Autodesk Inventor part; units mm, degrees
ref_plane "YZ Plane" through (0, 0, 0) normal (1, 0, 0) x (0, 1, 0)
ref_plane "XZ Plane" through (0, 0, 0) normal (0, 1, 0) x (-1, 0, 0)
ref_plane "XY Plane" through (0, 0, 0) normal (0, 0, 1) x (1, 0, 0)
sketch "Sketch1" plane through (0, 0, 0) normal (0, 0, 1) x (1, 0, 0)
  arc A0 (155.049, 9.8568) -> (142.3409, 9.8568) centre (148.6949, 9.8608) ccw
  circle A1 centre (148.6949, 9.8568) radius 2.1844
  circle A2 centre (148.6949, -15.5432) radius 2.1844
  line L0 (155.049, -4.0298) -> (155.049, 9.8568)
  arc A3 (155.049, -4.0298) -> (156.6938, -8.2941) centre (161.399, -4.0298) ccw
  arc A4 (145.4545, -25.8404) -> (156.6938, -8.2941) centre (148.6949, -15.5432) ccw
  arc A5 (135.9949, 3.5068) -> (142.3409, 9.8568) centre (135.9949, 9.8527) ccw
  line L1 (135.9949, 3.5068) -> (110.5949, 3.5068)
  arc A6 (104.2449, 9.8568) -> (110.5949, 3.5068) centre (110.5949, 9.8568) ccw
  line L2 (104.2449, 9.8568) -> (104.2449, 22.5568)
  circle A7 centre (97.8949, 9.8568) radius 2.1844
  circle A8 centre (97.8949, -2.8432) radius 2.1844
  circle A9 centre (97.8949, 22.5568) radius 2.1844
  circle A10 centre (-105.3051, 9.8568) radius 2.1844
  circle A11 centre (-105.3051, -2.8432) radius 2.1844
  circle A12 centre (-105.3051, 22.5568) radius 2.1844
  circle A13 centre (-156.1051, 9.8568) radius 2.1844
  circle A14 centre (-156.1051, -15.5432) radius 2.1844
  arc A15 (-164.1039, -8.2941) -> (-152.8646, -25.8404) centre (-156.1051, -15.5432) ccw
  line L3 (-162.4591, -4.0298) -> (-162.4591, 9.8568)
  arc A16 (-164.1039, -8.2941) -> (-162.4591, -4.0298) centre (-168.8091, -4.0298) ccw
  arc A17 (-149.751, 9.8568) -> (-162.4591, 9.8568) centre (-156.1051, 9.8608) ccw
  arc A18 (-149.751, 9.8568) -> (-143.4051, 3.5068) centre (-143.4051, 9.8527) ccw
  line L4 (-143.4051, 3.5068) -> (-118.0051, 3.5068)
  arc A19 (-118.0051, 3.5068) -> (-111.6551, 9.8568) centre (-118.0051, 9.8568) ccw
  line L5 (-111.6551, 9.8568) -> (-111.6551, 22.5568)
  circle A20 centre (-35.4551, 41.6068) radius 2.1844
  circle A21 centre (28.0449, 41.6068) radius 2.1844
  line L6 (-35.4551, 47.9568) -> (28.0449, 47.9568)
  line L7 (99.506, 28.699) -> (29.7157, 47.733)
  arc A22 (0.4819, 5.2197) -> (-7.892, 5.2197) centre (-3.7051, -6.7703) ccw
  arc A23 (40.7475, -8.8412) -> (42.841, -9.1962) centre (42.841, -2.8462) ccw
  line L8 (40.7475, -8.8412) -> (0.4819, 5.2197)
  arc A24 (-50.2511, -9.1962) -> (-48.1577, -8.8412) centre (-50.2511, -2.8462) ccw
  line L9 (-7.892, 5.2197) -> (-48.1577, -8.8412)
  arc A25 (104.2449, 22.5568) -> (99.506, 28.699) centre (97.8949, 22.5568) ccw
  line L10 (-106.9759, 28.683) -> (-37.1259, 47.733)
  arc A26 (-35.4551, 47.9568) -> (-37.1259, 47.733) centre (-35.4551, 41.6068) ccw
  arc A27 (29.7157, 47.733) -> (28.0449, 47.9568) centre (28.0449, 41.6068) ccw
  arc A28 (-106.9759, 28.683) -> (-111.6551, 22.5568) centre (-105.3051, 22.5568) ccw
  arc A29 (-96.072, -9.1962) -> (-103.6966, -10.3676) centre (-96.072, -34.5962) ccw
  arc A30 (96.2864, -10.3676) -> (88.6619, -9.1962) centre (88.6619, -34.5962) ccw
  line L11 (-103.6966, -10.3676) -> (-152.8646, -25.8404)
  line L12 (-96.072, -9.1962) -> (-50.2511, -9.1962)
  line L13 (88.6619, -9.1962) -> (42.841, -9.1962)
  line L14 (96.2864, -10.3676) -> (145.4545, -25.8404)
  point P0 (0, 0)
  dimension "d0" = 12.7
  dimension "d1" = 6.35
  dimension "d2" = 6.35
  dimension "d3" = 25.4
  dimension "d4" = 25.4
extrude "Extrusion1" add sketch "Sketch1" along normal blind 1.5875
properties part number "backaligner"
Could you check a few things on this model? Use its own coordinates, in mm. A direction names the side the tool comes from. Coordinates: 2 decimals unless noted, no trailing zeros. Write each loop counter-clockwise with the first axis right and the second up, starting at its lowest first coordinate (ties: lowest second). Pieces come first, ordered by that corner, then holes. Notation, with made-up numbers: (2, 85.25) -> (54, 85.25) arc R11 cw to (54, 101.25) -> close; hole circle Ø8 at (41.5, -39). An arc over 180 degrees is marked (long way). Write item = value, one per line. Start each with the question number.
(1) I want a section at A-A (z = 0.4). Give the number of separate pieces and of enclosed holes in the cut face, plus the area to 3 significant figures.
(2) I want a section at B-B (x = -21.5). Please give me the cut outline in (y, z).
(3) Which directions (+Z, -Z, +X, -X, +Y, -Y) give clear straight access to the entire face, cutting with the end or side of a thin tool? Please do faces 1 (the face through (106.15, 5.32, 0.78)), 2 (the face through (-127.936, -17.996, 0.783)), 3 (the face through (-6, 11, 0)).
(4) I need wall thicknesses on line 1 (X direction, y = 14, z = 0.5); line 2 (Y direction, x = 17, z = 1.2); line 3 (Y direction, x = 20, z = 1.4). Which ranges of each line are inside material? Lowest first, please. Write a range as [from, to].
(5) Will these pins go through, and if not, where does the flat tip stop? pin 1 (0.5 mm diameter, centred on x = 55, z = 0.5, fed in from -Y); pin 2 (0.5 mm diameter, centred on y = 18, z = 1, fed in from +X); pin 3 (0.8 mm diameter, centred on y = 3.5, z = 0.5, fed in from +X).
(6) I want a section at C-C (x = 36.5). Please give me the cut outline in (y, z).
(7) We'd pull the mould along X, two halves only. Please class faces 4 (the face through (120.526, -17.996, 0.783)), 5 (the face through (-6, 11, 1.588)), 6 (the face through (65.099, 38.083, 0.783)): released by +X, released by -X, zero draft, split by the parting line, or undercut.
Result set:
q1.separate_pieces = 1
q1.enclosed_holes = 12
q1.area = 12,800 mm2
q2.outline = (0.47, 0) -> (47.96, 0) -> (47.96, 1.59) -> (0.47, 1.59) -> close
q3.face_1 = +Z, -Z, +Y
q3.face_2 = +Z, -Z, -Y
q3.face_3 = -Z, +X, -X, +Y, -Y
q4.line_1 = [-160.93, -151.28], [-111.66, 104.24], [143.87, 153.52]
q4.line_2 = [-0.55, 47.96]
q4.line_3 = [-1.6, 47.96]
q5.pin_1 = -9.2
q5.pin_2 = 104.24
q5.pin_3 = 155.05
q6.outline = (-7.36, 0) -> (45.88, 0) -> (45.88, 1.59) -> (-7.36, 1.59) -> close
q7.face_4 = undercut
q7.face_5 = zero draft
q7.face_6 = released by +X
